Part print with two shaded views. Sizes in mm from the minimum x, y, z corner. Give positions to 0.01 mm unless a question says otherwise; leave off trailing zeros. Order: outer loops, then holes, each group sorted by start corner. A loop starts at its lowest first (then second) coordinate and runs counter-clockwise, first axis right, second up. Notation, with made-up numbers: (-23, 12.25) -> (15, 12.25) arc R31 cw to (15, 44.25) -> close; hole circle Ø4 at (28.5, -35). An arc over 180 degrees is marked (long way). Answer as CSV lines item,"result".
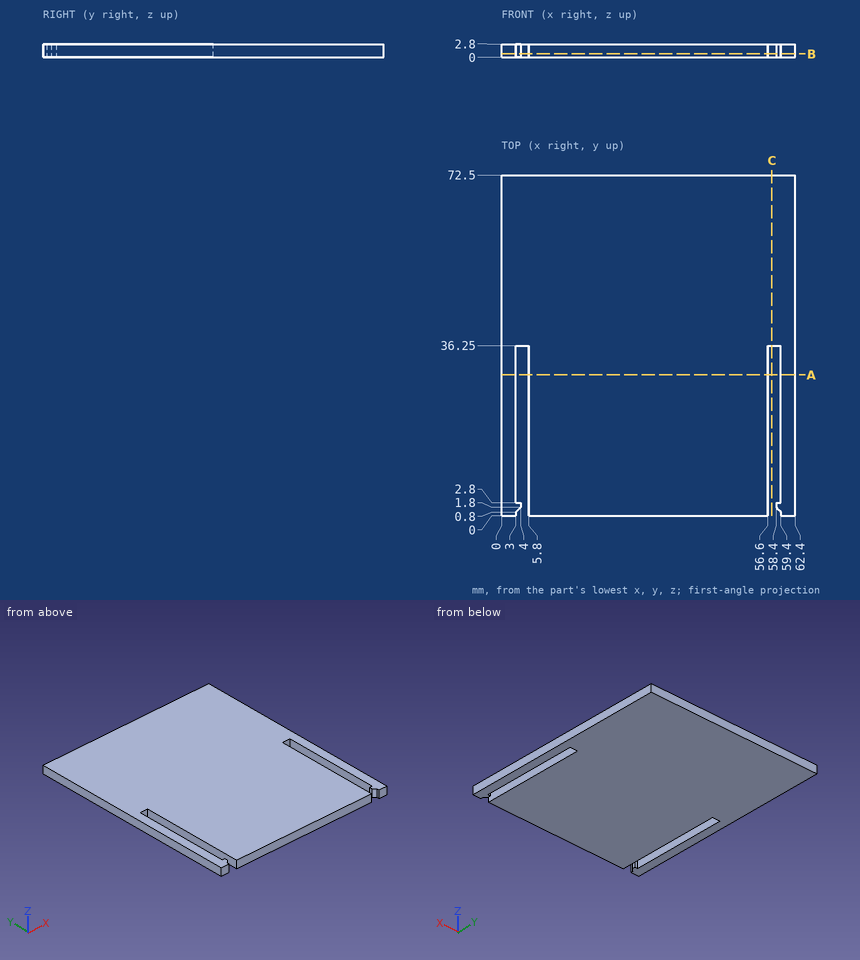
1) Band-saw the part on C-C, the plane x = 57.5. Write the cut outline in (y, z), then the cut area to 4 significant figures.
Data:
outline,"(36.25, 0) -> (72.5, 0) -> (72.5, 2.8) -> (36.25, 2.8) -> close"
area,"101.5 mm2"
2) Wall check: line 1 along X through (y, z) = (29.5, 2.15). Give the ranges that are in metal, low to high. Write a range as [from, to].
Data:
line 1,"x = [0, 3], [5.8, 56.6], [59.4, 62.4]"
3) Pin check, flat tip, straight feed: P1, Ø0.6, axis at y = 0.5, z = 1, coming from the -X side. Stop position of the tip, or through.
Data:
P1,"stops at x = 0"
4) Band-saw the part on A-A, the plane y = 30. Write the cut outline in (x, z).
Data:
outline,"(0, 0) -> (3, 0) -> (3, 2.8) -> (0, 2.8) -> close; (5.8, 0) -> (56.6, 0) -> (56.6, 2.8) -> (5.8, 2.8) -> close; (59.4, 0) -> (62.4, 0) -> (62.4, 2.8) -> (59.4, 2.8) -> close"
5) Band-saw the part on B-B, the plane z = 0.7. Write the cut outline in (x, y), then the cut area to 3 significant figures.
Data:
outline,"(0, 0) -> (3, 0) -> (3, 0.8) -> (4, 1.8) -> (4, 2.8) -> (3, 2.8) -> (3, 36.25) -> (5.8, 36.25) -> (5.8, 0) -> (56.6, 0) -> (56.6, 36.25) -> (59.4, 36.25) -> (59.4, 2.8) -> (58.4, 2.8) -> (58.4, 1.8) -> (59.4, 0.8) -> (59.4, 0) -> (62.4, 0) -> (62.4, 72.5) -> (0, 72.5) -> close"
area,"4,320 mm2"
